CAD build for the part. Positions are in the model's coordinates, mm. Face numbers are marked on the shaded views. A direction names the side the tool comes from. Coordinates: 2 decimals unless noted, no trailing zeros. Write each loop counter-clockwise with the first axis right and the second up, starting at its lowest first coordinate (ties: lowest second). Pieces come first, ordered by that corner, then holes. Notation, with made-up numbers: (48.5, 8.5) - (59.5, 8.5) arc R24 cw to (59.5, 22.5) - close; hole circle Ø9 at (41.5, 34.5). An arc over 180 degrees is marked (long way). Answer in a Markdown table with one row per item. Add a question column.
Q1. Band-saw the part on B-B (y = 9.5). List the corners of the cut face in (x, z).
Q2. Band-saw the part on C-C (z = 3.5). List the corners of the cut face in (x, y), and give its area (3 significant figures).
Q3. 3-axis set-ups, long thin cutter, end or side, ignore diameter. For the marked faces 1 and 2: which of +Z, -Z, +X, -X, +Y, -Y reach the whole face in a straight line?
Q4. Band-saw the part on D-D (x = 6). List the corners of the cut face in (y, z).
Q5. Drill centre lines: line 1 along X through (y, z) = (13, 3.15); line 2 along Y through (x, z) = (-23, 1.75); line 3 along Y through (x, z) = (24, 2.55). Where is each one in solid material? Low to high. Write a range as from..to.
Q6. Two-plate mould, pull along X, no slides. Class the marked faces 3, 4 and 5: +X half, -X half, draft (parallel to the pull), parting line (faces both ways), or undercut.
Q7. Band-saw the part on A-A (x = 0). List the corners of the cut face in (y, z).
Q8. Pin check, flat tip, straight feed: pin 1 (2 mm diameter, centred on x = 4, z = 4, fed in from -Y). Stop position of the tip, or through.
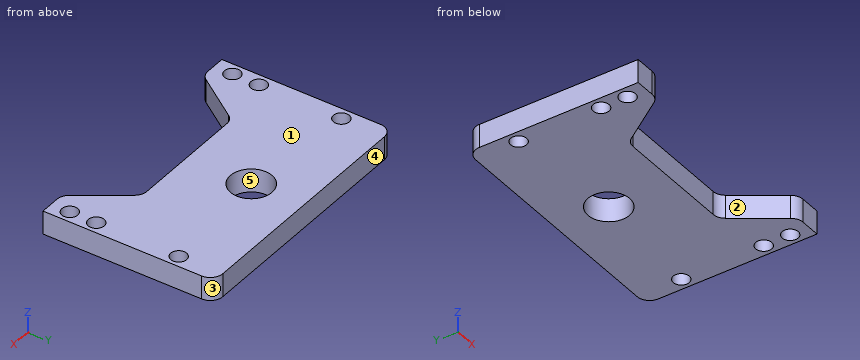
```python
from build123d import *

# Parameters (mm, degrees)
SKETCH1_R           = 1.63195
SKETCH1_R_2         = 4.245922678
BOSS_EXTRUDE1_DEPTH = 4.7625


with BuildPart() as part:
    # Sketch1 → Boss-Extrude1 (new body)
    with BuildSketch(Plane.XY):
        with BuildLine():
            Line((-26.26995, -11.1125), (-22.143527073, -11.1125))
            ThreePointArc((-22.143527073, -11.1125), (-20.967014102, -10.823592453), (-20.058141665, -10.022592307))
            Line((-20.058141665, -10.022592307), (-13.846715616, -1.089907693))
            ThreePointArc((-13.846715616, -1.089907693), (-12.937843178, -0.288907547), (-11.761330208, 0))
            Line((-11.761330208, 0), (11.761330208, 0))
            ThreePointArc((11.761330208, 0), (12.937843178, -0.288907547), (13.846715616, -1.089907693))
            Line((13.846715616, -1.089907693), (20.058141665, -10.022592307))
            ThreePointArc((20.058141665, -10.022592307), (20.967014102, -10.823592453), (22.143527073, -11.1125))
            Line((22.143527073, -11.1125), (26.26995, -11.1125))
            Line((26.26995, -11.1125), (26.26995, 21.2725))
            ThreePointArc((26.26995, 21.2725), (25.526001224, 23.068551224), (23.72995, 23.8125))
            Line((23.72995, 23.8125), (-23.72995, 23.8125))
            ThreePointArc((-23.72995, 23.8125), (-25.526001224, 23.068551224), (-26.26995, 21.2725))
            Line((-26.26995, 21.2725), (-26.26995, -11.1125))
        make_face()
        with Locations(Location((23.8887, 14.931889209, 0), (0, 0, 180))):
            Circle(SKETCH1_R, mode=Mode.SUBTRACT)
        with Locations(Location((23.8887, -7.293110791, 0), (0, 0, 180))):
            Circle(SKETCH1_R, mode=Mode.SUBTRACT)
        with Locations(Location((-23.8887, -7.293110791, 0), (0, 0, 180))):
            Circle(SKETCH1_R, mode=Mode.SUBTRACT)
        with Locations(Location((-23.8887, 14.931889209, 0), (0, 0, 180))):
            Circle(SKETCH1_R, mode=Mode.SUBTRACT)
        with Locations(Location((23.8887, -1.895610791, 0), (0, 0, 180))):
            Circle(SKETCH1_R, mode=Mode.SUBTRACT)
        with Locations(Location((-23.8887, -1.895610791, 0), (0, 0, 180))):
            Circle(SKETCH1_R, mode=Mode.SUBTRACT)
        with Locations(Location((0, 13.141292549, 0), (0, 0, 180))):
            Circle(SKETCH1_R_2, mode=Mode.SUBTRACT)
    extrude(amount=BOSS_EXTRUDE1_DEPTH)


solid = part.part
```
Checked values:
| question | item | result |
|---|---|---|
| 1 | outline | (-26.27, 0) - (-2.18, 0) - (-2.18, 4.76) - (-26.27, 4.76) - close; (2.18, 0) - (26.27, 0) - (26.27, 4.76) - (2.18, 4.76) - close |
| 2 | outline | (-26.27, -11.11) - (-22.14, -11.11) arc R2.54 ccw to (-20.06, -10.02) - (-13.85, -1.09) arc R2.54 cw to (-11.76, 0) - (11.76, 0) arc R2.54 cw to (13.85, -1.09) - (20.06, -10.02) arc R2.54 ccw to (22.14, -11.11) - (26.27, -11.11) - (26.27, 21.27) arc R2.54 ccw to (23.73, 23.81) - (-23.73, 23.81) arc R2.54 ccw to (-26.27, 21.27) - close; hole circle Ø3.26 at (-23.89, -7.29); hole circle Ø3.26 at (-23.89, -1.9); hole circle Ø3.26 at (-23.89, 14.93); hole circle Ø8.49 at (0, 13.14); hole circle Ø3.26 at (23.89, -7.29); hole circle Ø3.26 at (23.89, -1.9); hole circle Ø3.26 at (23.89, 14.93) |
| 2 | area | 1,350 mm² |
| 3 | face 1 | +Z, +X, -X, +Y, -Y |
| 3 | face 2 | +Z, -Z, -Y |
| 4 | outline | (0, 0) - (23.81, 0) - (23.81, 4.76) - (0, 4.76) - close |
| 5 | line 1 | x = -26.27..-4.24, 4.24..26.27 |
| 5 | line 2 | y = -11.11..-8.66, -5.92..-3.26, -0.53..13.56, 16.3..23.81 |
| 5 | line 3 | y = -11.11..-8.92, -5.66..-3.52, -0.27..13.3, 16.56..23.8 |
| 6 | face 3 | +X half |
| 6 | face 4 | draft |
| 6 | face 5 | undercut |
| 7 | outline | (0, 0) - (8.9, 0) - (8.9, 4.76) - (0, 4.76) - close; (17.39, 0) - (23.81, 0) - (23.81, 4.76) - (17.39, 4.76) - close |
| 8 | pin 1 | stops at y = 0 |
